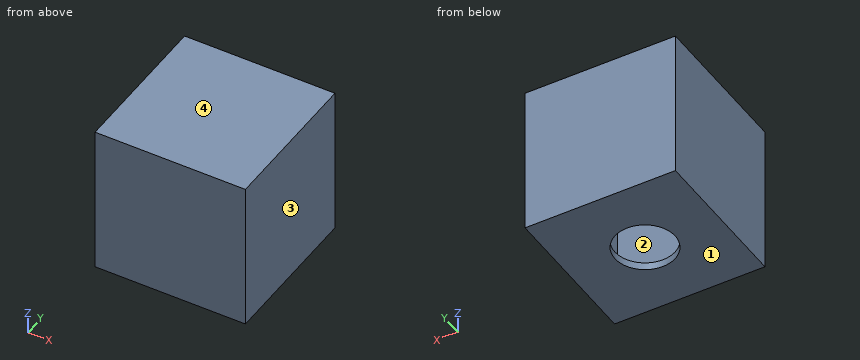
```python
from build123d import *

# Parameters (mm, degrees)
CYLINDER_R     = 100
CYLINDER_DEPTH = 50
BOX001_W       = 450
BOX001_H       = 450
BOX001_DEPTH   = 450
BOX013_W       = 500
BOX013_H       = 500
BOX013_DEPTH   = 500


with BuildPart() as cylinder:
    # Cylinder → Cylinder (new body)
    with BuildSketch(Plane(origin=(250, 250, -10), x_dir=(1, 0, 0), z_dir=(0, 0, 1))):
        Circle(CYLINDER_R)
    extrude(amount=CYLINDER_DEPTH)


with BuildPart() as cube001:
    # Box001 → Box001 (new body)
    with BuildSketch(Plane(origin=(25, 25, 25), x_dir=(1, 0, 0), z_dir=(0, 0, 1))):
        with Locations((225, 225)):
            Rectangle(BOX001_W, BOX001_H)
    extrude(amount=BOX001_DEPTH)


with BuildPart() as vacuumchamber:
    # Box013 → Box013 (new body)
    with BuildSketch(Plane.XY):
        with Locations((250, 250)):
            Rectangle(BOX013_W, BOX013_H)
    extrude(amount=BOX013_DEPTH)

    # Cut006: cut Cube001
    add(cube001.part, mode=Mode.SUBTRACT)

    # Cut001: cut Cylinder
    add(cylinder.part, mode=Mode.SUBTRACT)


solid = vacuumchamber.part
```
Verification items for the finished model (mm, model axes). Face numbers are marked on the shaded views. Round coordinates to 2 decimals unless told otherwise and drop trailing zeros. Write each loop counter-clockwise with the first axis right and the second up, starting at its lowest first coordinate (ties: lowest second). Pieces come first, ordered by that corner, then holes. Notation, with made-up numbers: (46, 54) - (76, 54) arc R9 cw to (76, 62) - close; hole circle Ø7 at (6, -35). An arc over 180 degrees is marked (long way). Answer as a JSON object with one key per item and string values. Group by question number.
Q1. Go/stop test with a flat-tipped pin: pin 1 Ø10 at (y, z) = (375.5, 283) entering from -X. Record where the tip stops, or that it passes through.
Q2. Section check C-C, the plane y = 250. Enter the section's corners in (x, z), plus the area to 3 significant figures.
Q3. Section check A-A, the plane x = 105. Enter the section's corners in (y, z), plus the area to 3 significant figures.
Q4. Mould release check, pull along Z, two halves, no side actions. Record for the marked faces 1, 2, 3 and 4: released by +Z, released by -Z, zero draft, split by the parting line, or undercut.
Q5. Thickness scan on line 1 (X direction, y = 250, z = 5); line 2 (Y direction, x = 316.5, z = 311.5). Record the ranges inside material, lowest first.
Found:
{
 "1": {"pin 1": "stops at x = 0"},
 "2": {"outline": "(0, 0) - (150, 0) - (150, 25) - (25, 25) - (25, 475) - (475, 475) - (475, 25) - (350, 25) - (350, 0) - (500, 0) - (500, 500) - (0, 500) - close", "area": "42,500 mm^2"},
 "3": {"outline": "(0, 0) - (500, 0) - (500, 500) - (0, 500) - close; hole (25, 25) - (475, 25) - (475, 475) - (25, 475) - close", "area": "47,500 mm^2"},
 "4": {"face 1": "released by -Z", "face 2": "undercut", "face 3": "zero draft", "face 4": "released by +Z"},
 "5": {"line 1": "x = 0 to 150, 350 to 500", "line 2": "y = 0 to 25, 475 to 500"}
}
